Geometry check sheet. Reference: the model listing, model coordinates, mm. A direction names the side the tool comes from. Give positions to 0.01 mm unless a question says otherwise; leave off trailing zeros. Write each loop counter-clockwise with the first axis right and the second up, starting at its lowest first coordinate (ties: lowest second). Pieces come first, ordered by that corner, then holes. Notation, with made-up numbers: (66, 72.25) - (125, 72.25) arc R17 ccw to (125, 80.25) - close; hole circle Ø10 at (-30, 15). An arc over 180 degrees is marked (long way). Use a Markdown table: item, result.
```python
from build123d import *

# Parameters (mm, degrees)
BOSS_EXTRUDE1_DEPTH = 3.175
FILLET1_R           = 1.5875
SKETCH3_R           = 0.79375
CUT_EXTRUDE1_DEPTH  = 3.175


with BuildPart() as part:
    # Sketch2 → Boss-Extrude1 (new body)
    with BuildSketch(Plane.XY):
        with BuildLine():
            Line((-19.05, 0), (-25.4, 0))
            Line((-25.4, 0), (0.767904, -19.675721))
            ThreePointArc((0.767904, -19.675721), (-4.290078, -10.020279), (0, 0))
            Line((0, 0), (-6.35, 0))
            Line((-6.35, 0), (-6.35, 3.175))
            Line((-6.35, 3.175), (-19.05, 3.175))
            Line((-19.05, 3.175), (-19.05, 0))
        make_face()
    extrude(amount=BOSS_EXTRUDE1_DEPTH)

    # Fillet1
    fillet1_edges = [part.edges().sort_by_distance(p)[0] for p in [
        (0.767904, -19.675721, 1.5875),
    ]]
    fillet(fillet1_edges, radius=FILLET1_R)

    # Sketch3 → Cut-Extrude1 (cut)
    with BuildSketch(Plane.XY.offset(3.175)):
        with Locations((-19.05, 0)):
            Circle(SKETCH3_R)
        with Locations((-6.35, 0)):
            Circle(SKETCH3_R)
    extrude(amount=-CUT_EXTRUDE1_DEPTH, mode=Mode.SUBTRACT)


solid = part.part
```
1) Material ranges on L1, parallel to X at y = 2, z = 2; L2, parallel to Y at x = -1.5, z = 0.75; L3, parallel to X at y = -3.5, z = 1, recorded low to high. Write a range as from..to.
Working result:
| item | result |
|---|---|
| L1 | x = -19.05..-6.35 |
| L2 | y = -1.57..0 |
| L3 | x = -20.75..-2.78 |
2) Depth check by flat-ended pin: P1, Ø1, axis at y = -1.5, z = 2.5, coming from the +X side; P2, Ø0.7, axis at y = 2.5, z = 1, coming from the -X side; P3, Ø1.9, axis at y = 2, z = 2, coming from the +X side. Enter the tip coordinate at first touch or a pass-through.
Working result:
| item | result |
|---|---|
| P1 | stops at x = -1.01 |
| P2 | stops at x = -19.05 |
| P3 | stops at x = -6.35 |
3) Section check C-C on y = -2. Record the boundary of the cut face in (x, z) (3 decimals).
Working result:
| item | result |
|---|---|
| outline | (-22.74, 0) - (-1.83, 0) - (-1.83, 3.175) - (-22.74, 3.175) - close |
4) Set-up check for faces 4 (the flat face through (-6.35, 2, 2)), 5 (the flat face through (-23, 0, 2)), 6 (the flat face through (-10, -4, 3.175)): record each of +Z, -Z, +X, -X, +Y, -Y from which the full face is reachable in a straight line by a thin tool's end or side.
Working result:
| item | result |
|---|---|
| face 4 | +Z, -Z, +X, +Y |
| face 5 | +Z, -Z, -X, +Y |
| face 6 | +Z, +X, -X, +Y, -Y |
5) Section check B-B on x = -2. Record the boundary of the cut face in (y, z) (3 decimals).
Working result:
| item | result |
|---|---|
| outline | (-2.236, 0) - (0, 0) - (0, 3.175) - (-2.236, 3.175) - close |
6) Mould release check, pull along X, two halves, no side actions. Record for faces 1 (the cylindrical face through (-18.51, -0.58, 1.61)), 2 (the flat face through (-10, -4, 0)), 3 (the cylindrical face through (-3.758, -5.855, 1.565)): pulls with the +X half, pulls with the -X half, needs draft (parallel to the pull), parting line crosses it, or undercut.
Working result:
| item | result |
|---|---|
| face 1 | undercut |
| face 2 | needs draft |
| face 3 | pulls with the +X half |
